```python
from build123d import *

# Parameters (mm, degrees)
SKETCH2_W           = 10
SKETCH2_H           = 160
BOSS_EXTRUDE1_DEPTH = 4.5
SKETCH3_W           = 10
SKETCH3_H           = 4.5
BOSS_EXTRUDE2_DEPTH = 20
FILLET1_R           = 5
FILLET2_R           = 5
FILLET3_R           = 5
CUT_EXTRUDE1_DEPTH  = 30
BOSS_EXTRUDE4_START = -20
SKETCH6_W           = 4.5
SKETCH6_H           = 10
BOSS_EXTRUDE4_DEPTH = 72


with BuildPart() as part:
    # Sketch2 → Boss-Extrude1 (new body)
    with BuildSketch(Plane(origin=(0, 0, 0), x_dir=(1, 0, 0), z_dir=(0, 1, 0))):
        with Locations((0, 93.515033533)):
            Rectangle(SKETCH2_W, SKETCH2_H)
    extrude(amount=BOSS_EXTRUDE1_DEPTH)

    # Sketch3 → Boss-Extrude2 (add)
    with BuildSketch(Plane(origin=(5, 0, 0), x_dir=(0, 0, -1), z_dir=(1, 0, 0))):
        with Locations((168.515033533, 2.25)):
            Rectangle(SKETCH3_W, SKETCH3_H)
    extrude(amount=BOSS_EXTRUDE2_DEPTH)

    # Fillet1
    fillet1_edges = [part.edges().sort_by_distance(p)[0] for p in [
        (5, 2.25, -163.515033533),
        (-5, 2.25, -173.515033533),
    ]]
    fillet(fillet1_edges, radius=FILLET1_R)

    # Fillet2
    fillet2_edges = [part.edges().sort_by_distance(p)[0] for p in [
        (-5, 2.25, -13.515033533),
        (5, 2.25, -13.515033533),
    ]]
    fillet(fillet2_edges, radius=FILLET2_R - 0.0001)  # a hair under: the kernel refuses the full size

    # Fillet3
    fillet3_edges = [part.edges().sort_by_distance(p)[0] for p in [
        (25, 2.25, -173.515033533),
        (25, 2.25, -163.515033533),
    ]]
    fillet(fillet3_edges, radius=FILLET3_R - 0.0001)  # a hair under: the kernel refuses the full size

    # Sketch4 → Cut-Extrude1 (cut)
    with BuildSketch(Plane(origin=(0, 4.5, 0), x_dir=(1, 0, 0), z_dir=(0, 1, 0))):
        with BuildLine():
            Line((-1.7, 18.515033533), (-1.7, 75.515033533))
            ThreePointArc((-1.7, 75.515033533), (0, 77.215033533), (1.7, 75.515033533))
            Line((1.7, 75.515033533), (1.7, 18.515033533))
            ThreePointArc((1.7, 18.515033533), (0, 16.815033533), (-1.7, 18.515033533))
        make_face()
        with BuildLine():
            Line((2, 166.515033533), (0, 166.515033533))
            ThreePointArc((0, 166.515033533), (-2, 168.515033533), (0, 170.515033533))
            Line((0, 170.515033533), (2, 170.515033533))
            ThreePointArc((2, 170.515033533), (4, 168.515033533), (2, 166.515033533))
        make_face()
        with BuildLine():
            Line((18, 170.515033533), (20, 170.515033533))
            ThreePointArc((20, 170.515033533), (22, 168.515033533), (20, 166.515033533))
            Line((20, 166.515033533), (18, 166.515033533))
            ThreePointArc((18, 166.515033533), (16, 168.515033533), (18, 170.515033533))
        make_face()
    extrude(amount=-CUT_EXTRUDE1_DEPTH, mode=Mode.SUBTRACT)

    # Sketch6 → Boss-Extrude4 (add)
    with BuildSketch(Plane(origin=(0, 0, -173.515033533), x_dir=(-1, 0, 0), z_dir=(0, 0, -1)).offset(BOSS_EXTRUDE4_START)):
        with Locations((0, 2.25)):
            Rectangle(SKETCH6_W, SKETCH6_H)
    extrude(amount=-BOSS_EXTRUDE4_DEPTH)


solid = part.part
```
Can you work these out from the model? Positions are in its coordinate system, mm. A direction names the side the tool comes from. Give positions to 0.01 mm unless a question says otherwise; leave off trailing zeros. Loops run counter-clockwise (first coordinate to the right, second up) from the corner with the lowest first, then second, coordinate; pieces in that order, holes last. Notation, with made-up numbers: M 65,4 L 79,4 A23 ccw 79,27 Z; hole C 21,9 d6. An arc over 180 degrees is marked long. Answer in a Markdown table with one row per item.
1. Suppose I cut it at B-B on y = 2.5. Count the separate pieces of the cut face and the enclosed holes in it, plus the area to 3 significant figures.
Taken from the geometry:
| item | result |
|---|---|
| separate pieces | 1 |
| enclosed holes | 3 |
| area | 1,530 mm² |
2. Suppose I cut it at D-D on x = 12.25. Write out the boundary of the cut face in (y, z), plus the area to 3 significant figures.
Taken from the geometry:
| item | result |
|---|---|
| outline | M 0,-173.52 L 4.5,-173.52 L 4.5,-163.52 L 0,-163.52 Z |
| area | 45.0 mm² |
3. Which directions (+Z, -Z, +X, -X, +Y, -Y) give clear straight access to the entire face, cutting with the end or side of a thin tool? Please do faces 5 (the cylindrical face through (0.037, 2.282, -16.815)), 6 (the flat face through (5, 2, -88)), 7 (the flat face through (-2.25, 6, -118)), 8 (the flat face through (0, -1, -153.515)), 9 (the flat face through (-2.25, -1, -118)).
Taken from the geometry:
| item | result |
|---|---|
| face 5 | +Y, -Y |
| face 6 | +Z, +X, +Y, -Y |
| face 7 | +Z, -Z, -X, +Y |
| face 8 | -Z, +X, -X, -Y |
| face 9 | +Z, -Z, -X, -Y |
4. Suppose I cut it at C-C on z = -94.5. Write out the boundary of the cut face in (x, y).
Taken from the geometry:
| item | result |
|---|---|
| outline | M -5,0 L -2.25,0 L -2.25,-2.75 L 2.25,-2.75 L 2.25,0 L 5,0 L 5,4.5 L 2.25,4.5 L 2.25,7.25 L -2.25,7.25 L -2.25,4.5 L -5,4.5 Z |
5. If I drill on line 1 along X through (y, z) = (2.25, -47); line 2 along Z through (x, y) = (19.5, 0.5); line 3 along X through (y, z) = (6.5, -152), over which ranges is the centre line in solid material (lowest first)?
Taken from the geometry:
| item | result |
|---|---|
| line 1 | x = -5 to -1.7, 1.7 to 5 |
| line 2 | z = -173.52 to -170.52, -166.52 to -163.52 |
| line 3 | x = -2.25 to 2.25 |
6. Suppose I cut it at A-A on z = -72.5. Write out the boundary of the cut face in (x, y).
Taken from the geometry:
| item | result |
|---|---|
| outline | M -5,0 L -1.7,0 L -1.7,4.5 L -5,4.5 Z; M 1.7,0 L 5,0 L 5,4.5 L 1.7,4.5 Z |
7. For pin 1 Ø5 at (x, y) = (19.5, -0.5) entering from +Z; pin 2 Ø2 at (y, z) = (1.5, -60) entering from +X; pin 3 Ø1.4 at (x, y) = (-1, -1.5) entering from +Z, each with a flat end and sliding along its axis, tell me the tip position at first contact or that it passes through.
Taken from the geometry:
| item | result |
|---|---|
| pin 1 | stops at z = -163.52 |
| pin 2 | stops at x = 5 |
| pin 3 | stops at z = -81.52 |
8. Thinking about a two-plate mould opening in X: for faces 1 (the flat face through (0, -1, -81.515)), 2 (the flat face through (-5, 2, -92)), 3 (the cylindrical face through (22, 2.3, -168.6)), 4 (the cylindrical face through (23.496, 2.282, -164.941)), which applies, released by +X, released by -X, zero draft, split by the parting line, or undercut?
Taken from the geometry:
| item | result |
|---|---|
| face 1 | zero draft |
| face 2 | released by -X |
| face 3 | undercut |
| face 4 | released by +X |
